For this review, take the finished solid that the model builds, in its own axes (mm). Face numbers are marked on the shaded views. A direction names the side the tool comes from. Coordinates: 2 decimals unless noted, no trailing zeros. Order: outer loops, then holes, each group sorted by start corner. A loop starts at its lowest first (then second) coordinate and runs counter-clockwise, first axis right, second up.
from build123d import *

# Parameters (mm, degrees)
SKETCH1_W           = 74
SKETCH1_H           = 59
BOSS_EXTRUDE1_DEPTH = 32
SHELL1_T            = -2
SKETCH2_R           = 5
CUT_EXTRUDE1_DEPTH  = 3


with BuildPart() as part:
    # Sketch1 → Boss-Extrude1 (new body)
    with BuildSketch(Plane(origin=(0, 0, 0), x_dir=(1, 0, 0), z_dir=(0, 1, 0))):
        Rectangle(SKETCH1_W, SKETCH1_H)
    extrude(amount=BOSS_EXTRUDE1_DEPTH)

    # Shell1
    shell1_openings = [part.faces().sort_by_distance(p)[0] for p in [
        (0, 32, 0),
    ]]
    offset(amount=SHELL1_T, openings=shell1_openings, kind=Kind.INTERSECTION)

    # Sketch2 → Cut-Extrude1 (cut)
    with BuildSketch(Plane(origin=(37, 0, 0), x_dir=(0, 0, -1), z_dir=(1, 0, 0))):
        with Locations((0, 16)):
            Circle(SKETCH2_R)
    extrude(amount=-CUT_EXTRUDE1_DEPTH, mode=Mode.SUBTRACT)


solid = part.part
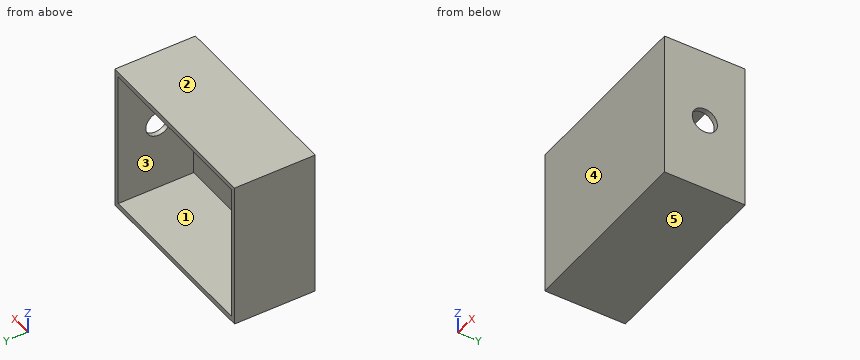
1. Take a section at C-C, the plane z = -21. Give the boundary of the cut face in (x, y).
Answer below:
outline: (-37, 0) - (37, 0) - (37, 32) - (35, 32) - (35, 2) - (-35, 2) - (-35, 32) - (-37, 32) - close
2. Take a section at B-B, the plane y = 16. Give the boundary of the cut face in (x, z).
Answer below:
outline: (-37, -29.5) - (37, -29.5) - (37, -5) - (35, -5) - (35, -27.5) - (-35, -27.5) - (-35, 27.5) - (35, 27.5) - (35, 5) - (37, 5) - (37, 29.5) - (-37, 29.5) - close
3. Machinability: for the marked faces 1 and 2, which of the approach directions +Z, -Z, +X, -X, +Y, -Y give a long, thin tool a straight path to every point of the face, cutting with its end or side? Answer none if there is none.
Answer below:
face 1: +Y
face 2: +Z, +X, -X, +Y, -Y
4. To check wall thickness, follow L1, parallel to X at y = 31, z = 9; L2, parallel to Z at x = 28, y = 19; L3, parallel to Y at x = 36, z = 0. State the ranges of each line that lie inside material, in increasing order.
Answer below:
L1: x = -37 to -35, 35 to 37
L2: z = -29.5 to -27.5, 27.5 to 29.5
L3: y = 0 to 11, 21 to 32
5. Take a section at D-D, the plane x = 18. Give the boundary of the cut face in (y, z), plus the area to 3 significant figures.
Answer below:
outline: (0, -29.5) - (32, -29.5) - (32, -27.5) - (2, -27.5) - (2, 27.5) - (32, 27.5) - (32, 29.5) - (0, 29.5) - close
area: 238 mm2
6. Clearance check with a flat-ended pin moving along its axis: pin 1 Ø6 at (y, z) = (16, 0) entering from +X. State where the tip first meets the part, or that it passes through.
Answer below:
pin 1: stops at x = -35
7. The part is to be moulded in two halves that separate along Z. For the marked faces 3, 4 and 5, say which applies: +Z half, -Z half, draft (parallel to the pull), parting line (faces both ways), or undercut.
Answer below:
face 3: undercut
face 4: draft
face 5: -Z half
8. Take a section at A-A, the plane z = 0. Give the boundary of the cut face in (x, y).
Answer below:
outline: (-37, 0) - (37, 0) - (37, 11) - (35, 11) - (35, 2) - (-35, 2) - (-35, 32) - (-37, 32) - close; (35, 21) - (37, 21) - (37, 32) - (35, 32) - close
